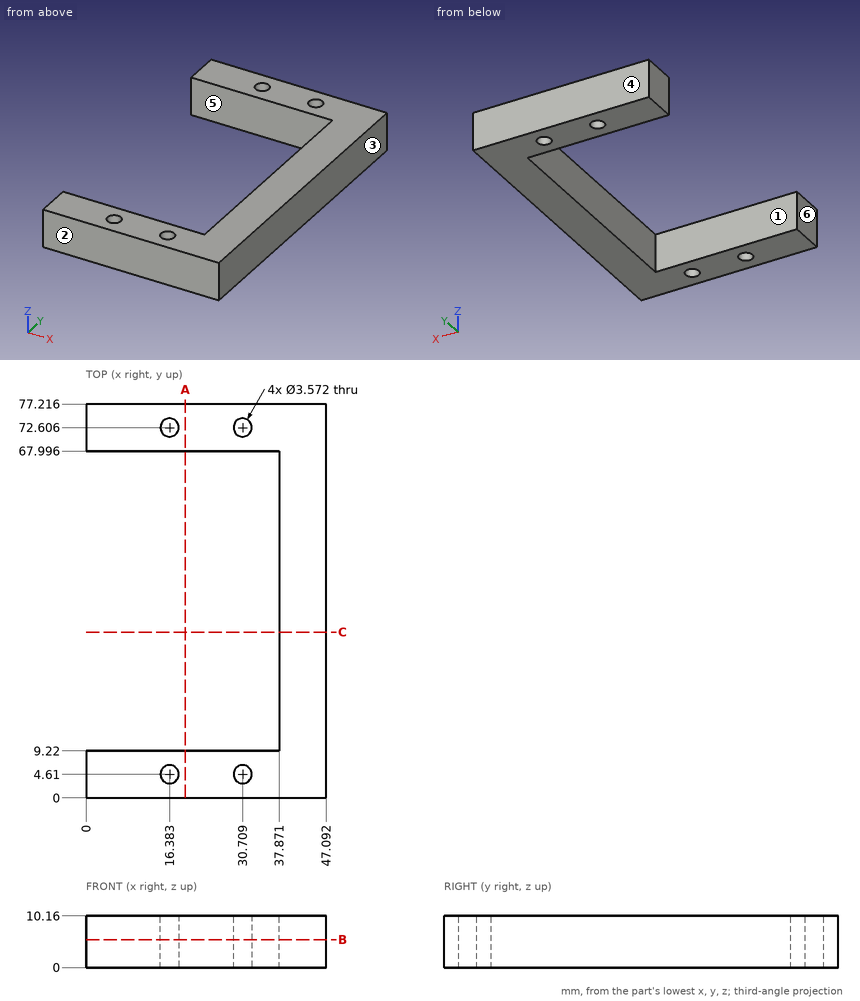
Design review of the part shown in the three views and the two pictorial views. Dimensions are in mm from the part's minimum x, y and z. A direction names the side the tool comes from. Round coordinates to 2 decimals unless told otherwise and drop trailing zeros. Write each loop counter-clockwise with the first axis right and the second up, starting at its lowest first coordinate (ties: lowest second). Pieces come first, ordered by that corner, then holes.
Item 1: The part is to be moulded in two halves that separate along Y. For the marked faces 1, 2, 3 and 4, say which applies: +Y half, -Y half, draft (parallel to the pull), parting line (faces both ways), or undercut.
Item 2: For the marked faces 5 and 6, list the 3-axis set-ups (+Z, -Z, +X, -X, +Y, -Y) from which the entire face can be reached by the end or side of a thin tool; tool diameter is ignored.
Item 3: We need section A-A on x = 19.5. Write out the cut boundary in (y, z) (1 decimal).
Item 4: We need section C-C on y = 32.5. Write out the cut boundary in (x, z).
Item 5: For probe 1 along Y at (x, z) = (25, 3) (1 decimal); probe 2 along X at (y, z) = (72.5, 6.5) (1 decimal); probe 3 along X at (y, z) = (37, 4.75), list the stretches that pass through material, from the lowest coordinate up.
Item 6: We need section B-B on z = 5.5. Write out the cut boundary in (x, y) (1 decimal).
Item 7: Clearance check with flat-ended pins moving along their axes: pin 1 Ø3 at (x, y) = (30.71, 4.61) entering from -Z; pin 2 Ø1.5 at (y, z) = (35.5, 7.5) entering from -X. State where each tip first meets the part, or that it passes through.
Returned:
1. face 1: undercut
1. face 2: -Y half
1. face 3: draft
1. face 4: +Y half
2. face 5: +Z, -Z, -X
2. face 6: +Z, -Z, -X, +Y, -Y
3. outline: (0, 0) - (9.2, 0) - (9.2, 10.2) - (0, 10.2) - close; (68, 0) - (77.2, 0) - (77.2, 10.2) - (68, 10.2) - close
4. outline: (37.87, 0) - (47.09, 0) - (47.09, 10.16) - (37.87, 10.16) - close
5. probe 1: y = 0 to 9.2, 68 to 77.2
5. probe 2: x = 0 to 14.6, 18.2 to 28.9, 32.5 to 47.1
5. probe 3: x = 37.87 to 47.09
6. outline: (0, 0) - (47.1, 0) - (47.1, 77.2) - (0, 77.2) - (0, 68) - (37.9, 68) - (37.9, 9.2) - (0, 9.2) - close; hole circle Ø3.6 at (16.4, 4.6); hole circle Ø3.6 at (16.4, 72.6); hole circle Ø3.6 at (30.7, 4.6); hole circle Ø3.6 at (30.7, 72.6)
7. pin 1: passes through
7. pin 2: stops at x = 37.87
